Can you work these out from the model? Positions are in its coordinate system, mm. Face numbers are marked on the shaded views. A direction names the side the tool comes from. Give positions to 0.01 mm unless a question says otherwise; leave off trailing zeros. Order: outer loops, then holes, each group sorted by start corner. A loop starts at its lowest first (then second) coordinate and runs counter-clockwise, first axis right, second up. Notation, with made-up numbers: (-7, 25.5) - (1, 25.5) arc R28 ccw to (1, 63.5) - close; hole circle Ø6 at (4, 25.25). An arc over 180 degrees is marked (long way). Use one line per item in the form item = value. Start each with the question number.
1) For pin 1 (1 mm diameter, centred on y = -2, z = 7, fed in from +X); pin 2 (0.6 mm diameter, centred on x = -1.5, y = 1.5, fed in from -Z); pin 3 (3 mm diameter, centred on y = -2.5, z = 13, fed in from +X), each with a flat end and sliding along its axis, tell me the tip position at first contact or that it passes through.
2) Please list where these lines run through material, in increasing order: probe 1 along Y at (x, z) = (-14, 9.5); probe 2 along X at (y, z) = (-6.5, -2); probe 3 along Z at (x, y) = (7, -1.25).
3) Suppose I cut it at A-A, the plane y = -2.5. Write out the boundary of the cut face in (x, z), and give its area (3 significant figures).
4) Suppose I cut it at D-D, the plane y = 1. Write out the boundary of the cut face in (x, z), and give its area (3 significant figures).
5) Suppose I cut it at B-B, the plane z = -7.5. Write out the boundary of the cut face in (x, y), and give its area (3 significant figures).
6) Which directions (+Z, -Z, +X, -X, +Y, -Y) give clear straight access to the entire face, cutting with the end or side of a thin tool? Please do the marked faces 1, 2 and 3.
7) Suppose I cut it at C-C, the plane x = -5. Write out the boundary of the cut face in (y, z).
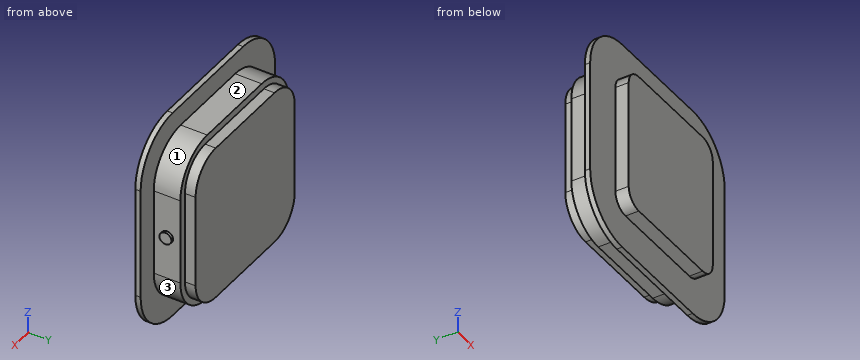
```python
from build123d import *

# Parameters (mm, degrees)
BOSS_EXTRUDE1_DEPTH = 2
BOSS_EXTRUDE2_DEPTH = 5
BOSS_EXTRUDE3_DEPTH = 1
BOSS_EXTRUDE4_DEPTH = 2.5
SKETCH5_R           = 1.127617125
BOSS_EXTRUDE5_DEPTH = 0.5


with BuildPart() as part:
    # Sketch1 → Boss-Extrude1 (new body)
    with BuildSketch(Plane(origin=(0, 0, 0), x_dir=(1, 0, 0), z_dir=(0, 1, 0))):
        with BuildLine():
            Line((8.732, -14.732), (-8.732, -14.732))
            ThreePointArc((-8.732, -14.732), (-12.974640687, -12.974640687), (-14.732, -8.732))
            Line((-14.732, -8.732), (-14.732, 8.732))
            ThreePointArc((-14.732, 8.732), (-12.974640687, 12.974640687), (-8.732, 14.732))
            Line((-8.732, 14.732), (8.732, 14.732))
            ThreePointArc((8.732, 14.732), (12.974640687, 12.974640687), (14.732, 8.732))
            Line((14.732, 8.732), (14.732, -8.732))
            ThreePointArc((14.732, -8.732), (12.974640687, -12.974640687), (8.732, -14.732))
        make_face()
    extrude(amount=BOSS_EXTRUDE1_DEPTH)

    # Sketch2 → Boss-Extrude2 (add)
    with BuildSketch(Plane.XZ):
        with BuildLine():
            Line((8.1, -16.122288114), (-8.1, -16.122288114))
            ThreePointArc((-8.1, -16.122288114), (-13.756854249, -13.779142364), (-16.1, -8.122288114))
            Line((-16.1, -8.122288114), (-16.1, 8.122288114))
            ThreePointArc((-16.1, 8.122288114), (-13.756854249, 13.779142364), (-8.1, 16.122288114))
            Line((-8.1, 16.122288114), (8.1, 16.122288114))
            ThreePointArc((8.1, 16.122288114), (13.756854249, 13.779142364), (16.1, 8.122288114))
            Line((16.1, 8.122288114), (16.1, -8.122288114))
            ThreePointArc((16.1, -8.122288114), (13.756854249, -13.779142364), (8.1, -16.122288114))
        make_face()
    extrude(amount=BOSS_EXTRUDE2_DEPTH)

    # Sketch3 → Boss-Extrude3 (add)
    with BuildSketch(Plane.XZ.offset(5)):
        with BuildLine():
            Line((10.47496, -20), (-10.47496, -20))
            ThreePointArc((-10.47496, -20), (-17.210152091, -17.210192091), (-19.99996, -10.475))
            Line((-19.99996, -10.475), (-19.99996, 10.475))
            ThreePointArc((-19.99996, 10.475), (-17.210152091, 17.210192091), (-10.47496, 20))
            Line((-10.47496, 20), (10.47496, 20))
            ThreePointArc((10.47496, 20), (17.210152091, 17.210192091), (19.99996, 10.475))
            Line((19.99996, 10.475), (19.99996, -10.475))
            ThreePointArc((19.99996, -10.475), (17.210152091, -17.210192091), (10.47496, -20))
        make_face()
    extrude(amount=BOSS_EXTRUDE3_DEPTH)

    # Sketch4 → Boss-Extrude4 (add)
    with BuildSketch(Plane.XZ.offset(6)):
        with BuildLine():
            Line((9.5, -13.25), (-9.5, -13.25))
            ThreePointArc((-9.5, -13.25), (-11.621320344, -12.371320344), (-12.5, -10.25))
            Line((-12.5, -10.25), (-12.5, 10.25))
            ThreePointArc((-12.5, 10.25), (-11.621320344, 12.371320344), (-9.5, 13.25))
            Line((-9.5, 13.25), (9.5, 13.25))
            ThreePointArc((9.5, 13.25), (11.621320344, 12.371320344), (12.5, 10.25))
            Line((12.5, 10.25), (12.5, -10.25))
            ThreePointArc((12.5, -10.25), (11.621320344, -12.371320344), (9.5, -13.25))
        make_face()
    extrude(amount=BOSS_EXTRUDE4_DEPTH)

    # Sketch5 → Boss-Extrude5 (add)
    with BuildSketch(Plane(origin=(16.1, 0, 0), x_dir=(0, 0, -1), z_dir=(1, 0, 0))):
        with Locations(Location((0, -2.5, 0), (0, 0, 180))):
            Circle(SKETCH5_R)
    extrude(amount=BOSS_EXTRUDE5_DEPTH)


solid = part.part
```
Result sheet:
q1.pin_1 = 16.1
q1.pin_2 = -14.73
q1.pin_3 = 15.35
q2.probe_1 = -6 to 2
q2.probe_2 = -12.5 to 12.5
q2.probe_3 = -16.12 to 16.12
q3.outline = (-16.1, -8.12) arc R8 ccw to (-8.1, -16.12) - (8.1, -16.12) arc R8 ccw to (16.1, -8.12) - (16.1, -1.13) - (16.6, -1.13) - (16.6, 1.13) - (16.1, 1.13) - (16.1, 8.12) arc R8 ccw to (8.1, 16.12) - (-8.1, 16.12) arc R8 ccw to (-16.1, 8.12) - close
q3.area = 984 mm²
q4.outline = (-14.73, -8.73) arc R6 ccw to (-8.73, -14.73) - (8.73, -14.73) arc R6 ccw to (14.73, -8.73) - (14.73, 8.73) arc R6 ccw to (8.73, 14.73) - (-8.73, 14.73) arc R6 ccw to (-14.73, 8.73) - close
q4.area = 837 mm²
q5.outline = (-20, -6) - (-12.5, -6) - (-12.5, -8.5) - (12.5, -8.5) - (12.5, -6) - (20, -6) - (20, -5) - (16.1, -5) - (16.1, 0) - (14.73, 0) - (14.73, 2) - (-14.73, 2) - (-14.73, 0) - (-16.1, 0) - (-16.1, -5) - (-20, -5) - close
q5.area = 322 mm²
q6.face_1 = +Z, +X, +Y
q6.face_2 = +Z, +X, -X, +Y
q6.face_3 = -Z, +X, +Y
q7.outline = (-8.5, -13.25) - (-6, -13.25) - (-6, -20) - (-5, -20) - (-5, -16.12) - (0, -16.12) - (0, -14.73) - (2, -14.73) - (2, 14.73) - (0, 14.73) - (0, 16.12) - (-5, 16.12) - (-5, 20) - (-6, 20) - (-6, 13.25) - (-8.5, 13.25) - close
